from build123d import *

# Parameters (mm, degrees)
F0_R     = 3.113344
F0_R_2   = 3.113341
F0_R_3   = 3.175
F0_R_4   = 3.113343
F1_DEPTH = 25.4


with BuildPart() as f1:
    # F0 (on Top) → F1 (new body)
    with BuildSketch(Plane.XY):
        with BuildLine():
            ThreePointArc((15.523532, -3.321986), (15.786888, -1.670264), (15.875, 0))
            ThreePointArc((15.875, 0), (15.670523, 2.539751), (15.062359, 5.014075))
            ThreePointArc((15.062359, 5.014075), (-1.498504, 15.804117), (-15.736312, 2.093829))
            ThreePointArc((-15.736312, 2.093829), (-15.862763, -0.623209), (-15.523539, -3.321951))
            ThreePointArc((-15.523539, -3.321951), (-1.8e-05, -15.875), (15.523532, -3.321986))
        make_face()
        Circle(F0_R, mode=Mode.SUBTRACT)
        with BuildLine():
            ThreePointArc((-15.736312, 2.093829), (-1.498504, 15.804117), (15.062359, 5.014075))
            Line((15.062359, 5.014075), (9.472198, 51.801542))
            ThreePointArc((9.472198, 51.801542), (9.51179, 51.301466), (9.525, 50.8))
            ThreePointArc((9.525, 50.8), (0.665006, 41.298243), (-9.432143, 49.473233))
            Line((-9.432143, 49.473233), (-15.736312, 2.093829))
        make_face()
        with Locations((-5.29085, 36.5252)):
            Circle(F0_R_2, mode=Mode.SUBTRACT)
        with BuildLine():
            Line((12.375646, -48.639175), (15.523532, -3.321986))
            ThreePointArc((15.523532, -3.321986), (-1.8e-05, -15.875), (-15.523539, -3.321951))
            Line((-15.523539, -3.321951), (-8.495912, -59.7936))
            ThreePointArc((-8.495912, -59.7936), (1.893103, -54.426187), (9.269192, -63.5))
            ThreePointArc((9.269192, -63.5), (7.414371, -69.062826), (2.592227, -72.399342))
            Line((2.592227, -72.399342), (44.631951, -71.435414))
            ThreePointArc((44.631951, -71.435414), (36.514353, -63.671517), (44.288918, -55.564135))
            Line((44.288918, -55.564135), (17.268347, -54.970898))
            ThreePointArc((17.268347, -54.970898), (13.617253, -52.735975), (12.375646, -48.639175))
        make_face()
        with BuildLine():
            ThreePointArc((9.525, 50.8), (9.51179, 51.301466), (9.472198, 51.801542))
            ThreePointArc((9.472198, 51.801542), (-1.164327, 60.253569), (-9.432143, 49.473233))
            ThreePointArc((-9.432143, 49.473233), (0.665006, 41.298243), (9.525, 50.8))
        make_face()
        with Locations((0, 50.8)):
            Circle(F0_R_3, mode=Mode.SUBTRACT)
        with BuildLine():
            ThreePointArc((9.269192, -63.5), (1.893103, -54.426187), (-8.495912, -59.7936))
            ThreePointArc((-8.495912, -59.7936), (-6.959853, -69.621958), (2.592227, -72.399342))
            ThreePointArc((2.592227, -72.399342), (7.414371, -69.062826), (9.269192, -63.5))
        make_face()
        with Locations((0, -63.5)):
            Circle(F0_R_3, mode=Mode.SUBTRACT)
        with BuildLine():
            Line((44.959223, -55.578851), (44.288918, -55.564135))
            ThreePointArc((44.288918, -55.564135), (36.514353, -63.671517), (44.631951, -71.435414))
            ThreePointArc((44.631951, -71.435414), (50.126625, -69.047958), (52.3875, -63.5))
            ThreePointArc((52.3875, -63.5), (50.239899, -58.070361), (44.959223, -55.578851))
        make_face()
        with Locations((44.45, -63.5)):
            Circle(F0_R_4, mode=Mode.SUBTRACT)
        with BuildLine():
            ThreePointArc((44.959223, -55.578851), (44.624226, -55.564412), (44.288918, -55.564135))
            Line((44.288918, -55.564135), (44.959223, -55.578851))
        make_face()
    extrude(amount=F1_DEPTH)


solid = f1.part
Geometry check sheet. Reference: the model listing, model coordinates, mm. A direction names the side the tool comes from. Round coordinates to 2 decimals unless told otherwise and drop trailing zeros. Loops run counter-clockwise (first coordinate to the right, second up) from the corner with the lowest first, then second, coordinate; pieces in that order, holes last. Notation, with made-up numbers: (78.25, 63) - (133.25, 63) arc R20 cw to (133.25, 69) - close; hole circle Ø5 at (-32.75, 18.5). An arc over 180 degrees is marked (long way). Answer as CSV lines item,"result".
(1) Cross-section at C-C, the plane z = 23.5. Give the number of separate pieces and of enclosed holes in the cut face, and give its area (3 significant figures).
Output values:
separate pieces,"1"
enclosed holes,"5"
area,"3,720 mm²"
(2) Cross-section at D-D, the plane y = -30.5. Enter the section's corners in (x, z).
Output values:
outline,"(-12.14, 0) - (13.64, 0) - (13.64, 25.4) - (-12.14, 25.4) - close"
(3) Depth check by flat-ended pin: pin 1 Ø10 at (y, z) = (25, 17) entering from -X; pin 2 Ø3 at (y, z) = (-34.5, 10.5) entering from +X; pin 3 Ø1.5 at (x, z) = (6, 7) entering from -Y. Enter the tip coordinate at first touch or a pass-through.
Output values:
pin 1,"stops at x = -13.35"
pin 2,"stops at x = 13.46"
pin 3,"stops at y = -72.34"
(4) Release check for a two-part mould opening along Y. For faces 3 (the face through (44.045, -60.413, 12.522)), 4 (the face through (-15.864, -0.585, 12.522)), 5 (the face through (15.676, 2.504, 12.522)) record: released by +Y, released by -Y, zero draft, split by the parting line, or undercut.
Output values:
face 3,"undercut"
face 4,"split by the parting line"
face 5,"released by +Y"
(5) Cross-section at A-A, the plane x = 0. Enter the section's corners in (y, z) (3 decimals).
Output values:
outline,"(-72.769, 0) - (-66.675, 0) - (-66.675, 25.4) - (-72.769, 25.4) - close; (-60.325, 0) - (-3.113, 0) - (-3.113, 25.4) - (-60.325, 25.4) - close; (3.113, 0) - (47.625, 0) - (47.625, 25.4) - (3.113, 25.4) - close; (53.975, 0) - (60.325, 0) - (60.325, 25.4) - (53.975, 25.4) - close"
(6) Cross-section at B-B, the plane x = 43. Enter the section's corners in (y, z).
Output values:
outline,"(-71.47, 0) - (-66.26, 0) - (-66.26, 25.4) - (-71.47, 25.4) - close; (-60.74, 0) - (-55.54, 0) - (-55.54, 25.4) - (-60.74, 25.4) - close"
(7) Material ranges on line 1 along Y through (x, z) = (0, 7.5) (3 decimals); line 2 along Y through (x, z) = (44.45, 5.75); line 3 along X through (y, z) = (38.5, 3), recorded low to high.
Output values:
line 1,"y = -72.769 to -66.675, -60.325 to -3.113, 3.113 to 47.625, 53.975 to 60.325"
line 2,"y = -71.44 to -66.61, -60.39 to -55.56"
line 3,"x = -10.89 to -7.7, -2.88 to 11.06"
(8) Set-up check for faces 1 (the face through (13.928, -26.298, 12.522)), 2 (the face through (12.306, 28.08, 12.522)): record each of +Z, -Z, +X, -X, +Y, -Y from which the full face is reachable in a straight line by a thin tool's end or side.
Output values:
face 1,"+Z, -Z, +X"
face 2,"+Z, -Z, +X, +Y"
